Input: part model. Units: mm. Frame: model coordinates. Face numbers are marked on the shaded views. A direction names the side the tool comes from. Give positions to 0.01 mm unless a question says otherwise; leave off trailing zeros. Loops run counter-clockwise (first coordinate to the right, second up) from the corner with the lowest first, then second, coordinate; pieces in that order, holes last. Notation, with made-up numbers: (25.25, 82) - (38.25, 82) arc R27 ccw to (38.25, 110) - close; hole circle Ø1 at (45, 85.25). An arc over 180 degrees is marked (long way). Answer as a JSON object with one key per item and string values.
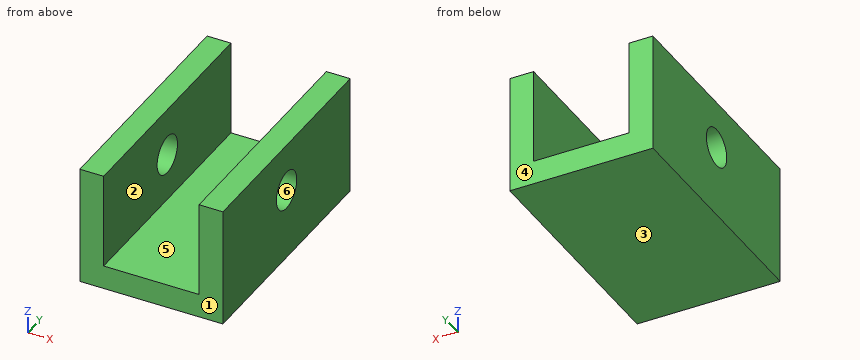
from build123d import *

# Parameters (mm, degrees)
SKETCH1_W           = 30
SKETCH1_H           = 50
BOSS_EXTRUDE1_DEPTH = 5
SKETCH2_W           = 5
SKETCH2_H           = 50
BOSS_EXTRUDE2_DEPTH = 20
SKETCH3_R           = 4
CUT_EXTRUDE1_DEPTH  = 47.368092477


with BuildPart() as part:
    # Sketch1 → Boss-Extrude1 (new body)
    with BuildSketch(Plane.XY):
        Rectangle(SKETCH1_W, SKETCH1_H)
    extrude(amount=BOSS_EXTRUDE1_DEPTH)

    # Sketch2 → Boss-Extrude2 (add)
    with BuildSketch(Plane.XY.offset(5)):
        with Locations((-12.5, 0)):
            Rectangle(SKETCH2_W, SKETCH2_H)
        with Locations((12.5, 0)):
            Rectangle(SKETCH2_W, SKETCH2_H)
    extrude(amount=BOSS_EXTRUDE2_DEPTH)

    # Sketch3 → Cut-Extrude1 (cut, through all)
    with BuildSketch(Plane(origin=(15, 0, 0), x_dir=(0, 0, -1), z_dir=(1, 0, 0))):
        with Locations((-15, 0)):
            Circle(SKETCH3_R)
    extrude(amount=-CUT_EXTRUDE1_DEPTH, mode=Mode.SUBTRACT)


solid = part.part
Item 1: Access query for the marked faces 1 and 2. Directions: +Z, -Z, +X, -X, +Y, -Y. A direction counts if a zero-diameter tool reaches every point of the face in a straight line with its end or side. Return the directions, or none.
Geometry check:
{"face 1": "+Z, -Z, +X, -X, -Y", "face 2": "+Z, +Y, -Y"}
Item 2: Cut plane A-A (y = 0). Return loops of the section in (x, z), then the cut area to 3 significant figures.
Geometry check:
{"outline": "(-15, 0) - (15, 0) - (15, 11) - (10, 11) - (10, 5) - (-10, 5) - (-10, 11) - (-15, 11) - close; (-15, 19) - (-10, 19) - (-10, 25) - (-15, 25) - close; (10, 19) - (15, 19) - (15, 25) - (10, 25) - close", "area": "270 mm2"}
Item 3: Cut plane B-B (z = 15). Return loops of the section in (x, y).
Geometry check:
{"outline": "(-15, -25) - (-10, -25) - (-10, -4) - (-15, -4) - close; (-15, 4) - (-10, 4) - (-10, 25) - (-15, 25) - close; (10, -25) - (15, -25) - (15, -4) - (10, -4) - close; (10, 4) - (15, 4) - (15, 25) - (10, 25) - close"}
Item 4: Cut plane C-C (z = 22). Return loops of the section in (x, y), then the cut area to 3 significant figures.
Geometry check:
{"outline": "(-15, -25) - (-10, -25) - (-10, 25) - (-15, 25) - close; (10, -25) - (15, -25) - (15, 25) - (10, 25) - close", "area": "500 mm2"}
Item 5: Mould query, pull axis Z, two halves, no side actions, for the marked faces 3, 4, 5 and 6. Classes: released by +Z, released by -Z, zero draft, split by the parting line, or undercut.
Geometry check:
{"face 3": "released by -Z", "face 4": "zero draft", "face 5": "released by +Z", "face 6": "undercut"}
Item 6: Material intervals for line 1 (X direction, y = -22.5, z = 14.75); line 2 (Y direction, x = 11.45, z = 15); line 3 (Z direction, x = -6, y = -17), sorted ascending. Write a range as [from, to].
Geometry check:
{"line 1": "x = [-15, -10], [10, 15]", "line 2": "y = [-25, -4], [4, 25]", "line 3": "z = [0, 5]"}
Item 7: Cut plane D-D (y = -17). Return loops of the section in (x, z), then the cut area to 3 significant figures.
Geometry check:
{"outline": "(-15, 0) - (15, 0) - (15, 25) - (10, 25) - (10, 5) - (-10, 5) - (-10, 25) - (-15, 25) - close", "area": "350 mm2"}
Item 8: Contact query for a flat-ended pin moving along its axis: P1, Ø5, axis at x = 4, y = 20, coming from the +Z side. Output: stop coordinate, or through.
Geometry check:
{"P1": "stops at z = 5"}
